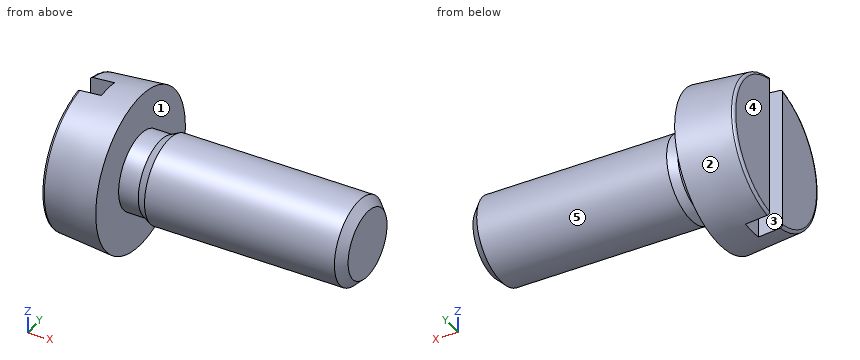
Autodesk Inventor part; units mm, degrees
ref_plane "Work Plane1" through (30.1625, 0, 0) normal (0, 0, -1) x (1, 0, 0)
ref_plane "YZ Plane" through (0, 0, 0) normal (1, 0, 0) x (0, 1, 0)
ref_plane "XZ Plane" through (0, 0, 0) normal (0, 1, 0) x (-1, 0, 0)
sketch "Sketch1" plane through (0, 0, 0) normal (0, 0, 1) x (1, 0, 0)
  line L0 (-2, 0) -> (8, 0)
  line L1 (8, 0) -> (8, 1.5)
  line L2 (8, 1.5) -> (1, 1.5)
  line L3 (1, 1.5) -> (0.6932, 1.3467)
  line L4 (0.6932, 1.3467) -> (0, 1.3467)
  line L5 (0, 1.3467) -> (0, 2.75)
  line L6 (-4, 0) -> (10, 0)
  line L7 (0, -0.55) -> (0, 3.3)
  line L8 (-2, 0) -> (-2, 2.575)
  line L9 (0, 2.75) -> (-2, 2.575)
  line L10 (1, 1.5) -> (0, 1.5) construction
  dimension "d0" = 8
  dimension "d1" = 7
  dimension "d2" = 0.3068
  dimension "d3" = 2
  dimension "d4" = 3
  dimension "d5" = 2.6935
  dimension "d9" = 5.5
  dimension "d10" = 5
revolve "Body" add sketch "Sketch1" angle 360 about axis through (-2, 0, 0) along (1, 0, 0)
sketch "Sketch2" plane through (-2, 0, 0) normal (-1, 0, 0) x (0, 0, 1)
  circle A0 centre (0, 0) radius 2.75
  line L0 (0, 0) -> (0, 2.575)
  line L1 (-2.75, 0.4) -> (2.75, 0.4)
  line L2 (2.75, 0.4) -> (2.75, -0.4)
  line L3 (2.75, -0.4) -> (-2.75, -0.4)
  line L4 (-2.75, -0.4) -> (-2.75, 0.4)
  line L5 (-2.75, 0) -> (2.75, 0) construction
  line L6 (0, 0.4) -> (0, -0.4) construction
  dimension "d11" = 0.8
  dimension "d12" = 5.5
fillet "Fillet1" radius 0.1 1 edges at (-2, -2.575, 0)
extrude "Slot" cut sketch "Sketch2" against normal blind 0.85 contours A0 L3 L1 | L2 L3 A0 | A0 L1 L2 | A0 L4 L1 | L3 L4 A0
thread "Thread"
chamfer "Chamfer1" distance 0.3067 distance2 0.3068 1 edges at (8, -1.5, 0) measured on face at (8, 0.417, 0.2189)
ref_plane "Work Plane1" through (30.1625, 0, 0) normal (0, 0, -1) x (1, 0, 0)
equation "\"d11\" = SBR"
equation "\"d12\" = KOD"
equation "\"d19\" = STI"
equation "\"d14\" = RR"
equation "\"d15\" = GEL"
equation "\"d17\" = -0.5 * SPD + 0.5 * GD"
equation "\"d0\" = NLG"
equation "\"d1\" = GEL"
equation "\"d3\" = KOH"
equation "\"d4\" = GD"
equation "\"d5\" = BDM"
equation "\"d9\" = KOD"
equation "\"d10\" = KEWI"
equation "\"GD\" = NND"
equation "\"NLG\" = 8"
equation "\"GEL\" = 7"
equation "\"KOD\" = 5.5"
equation "\"KOH\" = 2"
equation "\"GAL\" = 0.61345 * PTC"
equation "\"SPD\" = NND - 1.2269 * PTC"
equation "\"BDM\" = 2.6935"
equation "\"GUL\" = 0.61345 * PTC"
equation "\"RR\" = 0.1"
equation "\"SBR\" = 0.8"
equation "\"STI\" = 0.85"
equation "\"KEWI\" = 5deg"
equation "\"PTC\" = 0.5"
equation "\"THREADDIA\" = 3"
equation "\"TOA\" = 30deg"
equation "\"NND\" = 3"
equation "\"GD1\" = THREADDIA - 1.2269 * PTC"
properties part number "ISO 1207 - M3 x 8" material "Stainless Steel, 440C"
Design review of the part built by this model. Coordinates are the model's own, in mm. Face numbers are marked on the shaded views. A direction names the side the tool comes from. Give positions to 0.01 mm unless a question says otherwise; leave off trailing zeros. Order: outer loops, then holes, each group sorted by start corner. A loop starts at its lowest first (then second) coordinate and runs counter-clockwise, first axis right, second up. Notation, with made-up numbers: (-18.5, 17) -> (4.5, 17) arc R13 ccw to (4.5, 25) -> close; hole circle Ø4 at (19.5, 79). An arc over 180 degrees is marked (long way). Write item = value, one per line. Start each with the question number.
(1) For pin 1 (0.7 mm diameter, centred on x = -1.5, z = 0.5, fed in from -Y); pin 2 (0.7 mm diameter, centred on x = -1.5, z = 0.5, fed in from +Y); pin 3 (1.6 mm diameter, centred on y = -1.5, z = -1.5, fed in from +X), all flat-tipped, find the tip position at first contact; note any pin that passes through.
(2) We need section C-C on x = 1.5. Write out the cut boundary in (y, z).
(3) For the marked faces 1 and 2, list the 3-axis set-ups (+Z, -Z, +X, -X, +Y, -Y) from which the entire face can be reached by the end or side of a thin tool; tool diameter is ignored.
(4) To check wall thickness, follow line 1 along X through (y, z) = (1.1, 1.3); line 2 along X through (y, z) = (-0.05, 2.05); line 3 along Y through (x, z) = (6.5, -1.15). State the ranges of each line that lie inside material, in increasing order.
(5) We need section A-A on z = 0. Write out the cut boundary in (x, y).
(6) We need section B-B on y = 0. Write out the cut boundary in (x, z).
(7) Mouldability with a two-part tool opening along Y and no side actions: class the marked faces 3, 4 and 5 as +Y half, -Y half, draft (parallel to the pull), parting line (faces both ways), or undercut.
Numbers:
q1.pin_1 = -2.63
q1.pin_2 = 2.63
q1.pin_3 = 7.87
q2.outline = circle Ø3 at (0, 0)
q3.face_1 = none
q3.face_2 = -X
q4.line_1 = -2 to 0
q4.line_2 = -1.15 to 0
q4.line_3 = -0.96 to 0.96
q5.outline = (-2, -2.48) arc R0.1 ccw to (-1.91, -2.58) -> (0, -2.75) -> (0, -1.35) -> (0.69, -1.35) -> (1, -1.5) -> (7.69, -1.5) -> (8, -1.19) -> (8, 1.19) -> (7.69, 1.5) -> (1, 1.5) -> (0.69, 1.35) -> (0, 1.35) -> (0, 2.75) -> (-1.91, 2.58) arc R0.1 ccw to (-2, 2.48) -> (-2, 0.4) -> (-1.15, 0.4) -> (-1.15, -0.4) -> (-2, -0.4) -> close
q6.outline = (-1.15, -2.65) -> (0, -2.75) -> (0, -1.35) -> (0.69, -1.35) -> (1, -1.5) -> (7.69, -1.5) -> (8, -1.19) -> (8, 1.19) -> (7.69, 1.5) -> (1, 1.5) -> (0.69, 1.35) -> (0, 1.35) -> (0, 2.75) -> (-1.15, 2.65) -> close
q7.face_3 = undercut
q7.face_4 = draft
q7.face_5 = parting line
